```python
from build123d import *

# Parameters (mm, degrees)
SKETCH1_W           = 25.4
SKETCH1_H           = 25.4
SKETCH1_W_2         = 22.225
SKETCH1_H_2         = 22.225
BOSS_EXTRUDE1_DEPTH = 215.9
SKETCH2_R           = 4
SKETCH2_R_2         = 4.7625
SKETCH2_R_3         = 3.175
CUT_EXTRUDE1_DEPTH  = 218.759638133
SKETCH3_R           = 3.175
CUT_EXTRUDE2_DEPTH  = 218.759638133
SKETCH5_R           = 1.25
CUT_EXTRUDE3_DEPTH  = 218.759638133


with BuildPart() as part:
    # Sketch1 → Boss-Extrude1 (new body)
    with BuildSketch(Plane(origin=(0, 0, 0), x_dir=(1, 0, 0), z_dir=(0, 1, 0))):
        Rectangle(SKETCH1_W, SKETCH1_H)
        Rectangle(SKETCH1_W_2, SKETCH1_H_2, mode=Mode.SUBTRACT)
    extrude(amount=BOSS_EXTRUDE1_DEPTH)

    # Sketch2 → Cut-Extrude1 (cut, through all)
    with BuildSketch(Plane.XY.offset(12.7)):
        with Locations((0, 88.9)):
            Circle(SKETCH2_R)
        with Locations((0, 165.1)):
            Circle(SKETCH2_R_2)
        with Locations((0, 12.7)):
            Circle(SKETCH2_R_2)
        with Locations((0, 203.2)):
            Circle(SKETCH2_R_3)
    extrude(amount=-CUT_EXTRUDE1_DEPTH, mode=Mode.SUBTRACT)

    # Sketch3 → Cut-Extrude2 (cut, through all)
    with BuildSketch(Plane.XY.offset(12.7)):
        with Locations((3.302, 38.1)):
            Circle(SKETCH3_R)
    extrude(amount=-CUT_EXTRUDE2_DEPTH, mode=Mode.SUBTRACT)

    # Sketch5 → Cut-Extrude3 (cut, through all)
    with BuildSketch(Plane.ZY.offset(12.7)):
        with Locations((0, 43.6)):
            Circle(SKETCH5_R)
        with Locations((0, 29.6)):
            Circle(SKETCH5_R)
    extrude(amount=-CUT_EXTRUDE3_DEPTH, mode=Mode.SUBTRACT)


solid = part.part
```
Can you work these out from the model? Positions are in its coordinate system, mm. A direction names the side the tool comes from. Round coordinates to 2 decimals unless told otherwise and drop trailing zeros. Loops run counter-clockwise (first coordinate to the right, second up) from the corner with the lowest first, then second, coordinate; pieces in that order, holes last. Notation, with made-up numbers: (4.25, 5) -> (57.25, 5) arc R10 cw to (57.25, 13) -> close; hole circle Ø5 at (-22.5, -4.75). An arc over 180 degrees is marked (long way). Answer in a Markdown table with one row per item.
Item 1: We'd pull the mould along Y, two halves only. Please class faces 3 (the flat face through (0, 106, 12.7)), 4 (the cylindrical face through (-1.03, 8.05, 11.92)), 5 (the flat face through (-11.3, 0, -0.1)): released by +Y, released by -Y, zero draft, split by the parting line, or undercut.
Answer block:
| item | result |
|---|---|
| face 3 | zero draft |
| face 4 | undercut |
| face 5 | released by -Y |
Item 2: If I drill on probe 1 along Y at (x, z) = (12.1, 0); probe 2 along X at (y, z) = (81, -2.5); probe 3 along X at (y, z) = (203.2, 12) (3 decimals), over which ranges is the centre line in solid material (lowest first)?
Answer block:
| item | result |
|---|---|
| probe 1 | 0 to 28.35, 30.85 to 42.35, 44.85 to 215.9 |
| probe 2 | -12.7 to -11.11, 11.11 to 12.7 |
| probe 3 | -12.7 to -3.175, 3.175 to 12.7 |
Item 3: Will this pin go through, and if not, where does the flat tip stop? P1, Ø4, axis at y = 43.6, z = 0, coming from the -X side.
Answer block:
| item | result |
|---|---|
| P1 | x = -12.7 |
Item 4: On a 3-axis mill with a long thin cutter (end or side, diameter ignored), from which of +Z, -Z, +X, -X, +Y, -Y can I reach the whole of each face in a straight line? I mean faces 1 (the cylindrical face through (1.846, 85.351, 11.917)), 2 (the flat face through (0, 106, 11.112)). Say none if no direction works.
Answer block:
| item | result |
|---|---|
| face 1 | +Z, -Z |
| face 2 | +Y, -Y |
Item 5: Suppose I cut it at A-A, the plane y = 203.2. List the corners of the cut face in (x, z) for me (1 decimal).
Answer block:
| item | result |
|---|---|
| outline | (-12.7, -12.7) -> (-3.2, -12.7) -> (-3.2, -11.1) -> (-11.1, -11.1) -> (-11.1, 11.1) -> (-3.2, 11.1) -> (-3.2, 12.7) -> (-12.7, 12.7) -> close; (3.2, -12.7) -> (12.7, -12.7) -> (12.7, 12.7) -> (3.2, 12.7) -> (3.2, 11.1) -> (11.1, 11.1) -> (11.1, -11.1) -> (3.2, -11.1) -> close |
Item 6: Suppose I cut it at C-C, the plane x = -8.25. List the corners of the cut face in (y, z) for me, plus the area to 3 significant figures.
Answer block:
| item | result |
|---|---|
| outline | (0, -12.7) -> (215.9, -12.7) -> (215.9, -11.11) -> (0, -11.11) -> close; (0, 11.11) -> (215.9, 11.11) -> (215.9, 12.7) -> (0, 12.7) -> close |
| area | 685 mm² |
Item 7: Suppose I cut it at B-B, the plane z = -5.5. List the corners of the cut face in (x, y) for me.
Answer block:
| item | result |
|---|---|
| outline | (-12.7, 0) -> (-11.11, 0) -> (-11.11, 215.9) -> (-12.7, 215.9) -> close; (11.11, 0) -> (12.7, 0) -> (12.7, 215.9) -> (11.11, 215.9) -> close |
Item 8: Suppose I cut it at D-D, the plane y = 78. List the corners of the cut face in (x, z) for me.
Answer block:
| item | result |
|---|---|
| outline | (-12.7, -12.7) -> (12.7, -12.7) -> (12.7, 12.7) -> (-12.7, 12.7) -> close; hole (-11.11, -11.11) -> (11.11, -11.11) -> (11.11, 11.11) -> (-11.11, 11.11) -> close |
